The drawing under review shows one solid part. Ordinate dimensions are in mm from its lowest x, y, z. Coordinates: 2 decimals unless noted, no trailing zeros. Write each loop counter-clockwise with the first axis right and the second up, starting at its lowest first coordinate (ties: lowest second). Pieces come first, ordered by that corner, then holes.
Q1. For probe 1 along Y at (x, z) = (8, 4.5); probe 2 along X at (y, z) = (8, 5.25); probe 3 along Y at (x, z) = (5.75, 2.75), list the stretches that pass through material, from the lowest coordinate up.
Q2. Take a section at B-B (y = 4.5). Give the boundary of the cut face in (x, z).
Q3. Take a section at C-C (y = 8). Give the boundary of the cut face in (x, z).
Q4. Take a section at D-D (x = 3.25). Give the boundary of the cut face in (y, z).
Q5. Insertion check: pin 1 (6 mm diameter, centred on x = 6.5, z = 6, fed in from +Y); pin 2 (4 mm diameter, centred on x = 13, z = 6.5, fed in from -Y); pin 3 (3 mm diameter, centred on x = 14.5, z = 4.5, fed in from +Y); pin 4 (1.5 mm diameter, centred on x = 4.5, y = 3.5, fed in from -Z). Each pin has a flat end and moves straight along its axis. Give the tip position at first contact, or say it passes through.
Q6. Take a section at A-A (x = 8). Give the boundary of the cut face in (y, z), and give its area (3 significant figures).
Q7. Mouldability with a two-part tool opening along Y and no side actions: class the marked faces 1, 2, 3 and 4 as pulls with the +Y half, pulls with the -Y half, needs draft (parallel to the pull), parting line crosses it, or undercut.
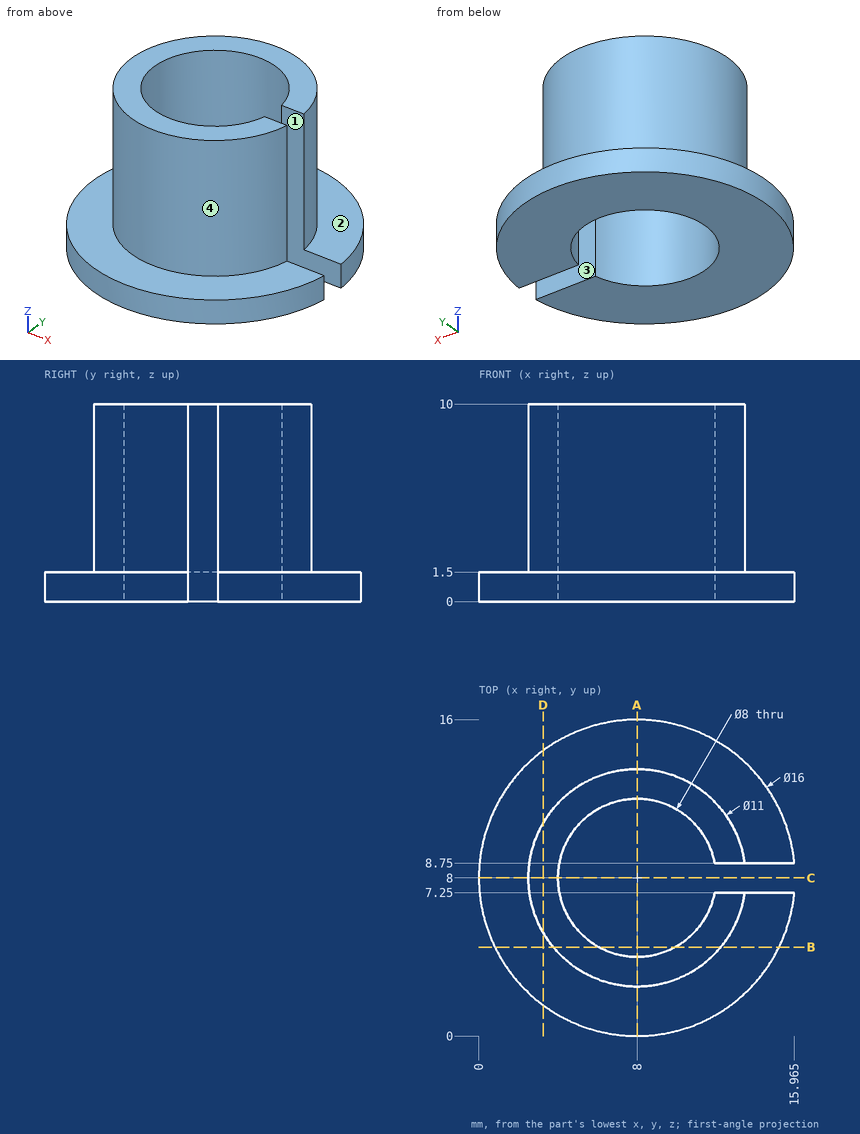
Response:
1. probe 1: y = 2.5 to 4, 12 to 13.5
1. probe 2: x = 2.5 to 4
1. probe 3: y = 2.98 to 4.69, 11.31 to 13.02
2. outline: (0.81, 0) - (6.06, 0) - (6.06, 10) - (3.76, 10) - (3.76, 1.5) - (0.81, 1.5) - close; (9.94, 0) - (15.19, 0) - (15.19, 1.5) - (12.24, 1.5) - (12.24, 10) - (9.94, 10) - close
3. outline: (0, 0) - (4, 0) - (4, 10) - (2.5, 10) - (2.5, 1.5) - (0, 1.5) - close
4. outline: (1.56, 0) - (14.44, 0) - (14.44, 1.5) - (10.77, 1.5) - (10.77, 10) - (5.23, 10) - (5.23, 1.5) - (1.56, 1.5) - close
5. pin 1: stops at y = 13.5
5. pin 2: stops at y = 3.39
5. pin 3: stops at y = 10.29
5. pin 4: stops at z = 0
6. outline: (0, 0) - (4, 0) - (4, 10) - (2.5, 10) - (2.5, 1.5) - (0, 1.5) - close; (12, 0) - (16, 0) - (16, 1.5) - (13.5, 1.5) - (13.5, 10) - (12, 10) - close
6. area: 37.5 mm2
7. face 1: undercut
7. face 2: needs draft
7. face 3: undercut
7. face 4: parting line crosses it
